Build history of the part. All positions in model axes, mm. Give positions to 0.01 mm unless a question says otherwise; leave off trailing zeros. Order: outer loops, then holes, each group sorted by start corner. A loop starts at its lowest first (then second) coordinate and runs counter-clockwise, first axis right, second up. Notation, with made-up numbers: (53, -13.5) - (58, -13.5) arc R12 cw to (58, 6.5) - close; hole circle Ø10 at (-29, 23.25). An arc over 180 degrees is marked (long way). Answer in a Markdown table with one row per item.
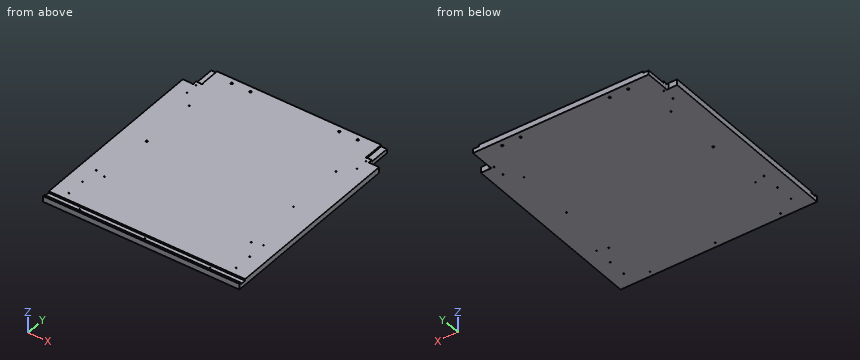
```python
from build123d import *

# Parameters (mm, degrees)
CABBACK_THICKNESS_DEPTH = 17.78
SKETCH4_R               = 3.175000003
SKETCH4_R_2             = 3.175000002
CUT_EXTRUDE1_DEPTH      = 17.78
SKETCH6_R               = 1.5875
SKETCH6_R_2             = 1.587500002
SKETCH6_R_3             = 2.777849083
CUT_EXTRUDE3_DEPTH      = 17.78
CABBACK_LEDGECUTS_W     = 17.78
CABBACK_LEDGECUTS_H     = 63.5
LEDGECUTS_DEPTH_DEPTH   = 5.08
SKETCH7_R               = 3.302
SKETCH7_R_2             = 3.302000002
CUT_EXTRUDE4_DEPTH      = 5.08
SKETCH9_R               = 3.175
CUT_EXTRUDE5_DEPTH      = 17.78


with BuildPart() as part:
    # CabBack_Outline → CabBack_Thickness (new body)
    with BuildSketch(Plane.XY):
        Polygon((10806.641666666, -6342.0625), (11409.891666666, -6342.0625), (11409.891666666, -5755.3225), (11378.141666665, -5755.3225), (11378.141666665, -5679.1225), (10838.391666667, -5679.1225), (10838.391666667, -5755.3225), (10806.641666666, -5755.3225), align=None)
    extrude(amount=-CABBACK_THICKNESS_DEPTH)

    # Sketch4 → Cut-Extrude1 (cut)
    with BuildSketch(Plane.XY):
        with Locations((11380.386730695, -5753.07743597)):
            Circle(SKETCH4_R)
        with Locations((10836.146602637, -5753.07743597)):
            Circle(SKETCH4_R_2)
    extrude(amount=-CUT_EXTRUDE1_DEPTH, mode=Mode.SUBTRACT)

    # Sketch6 → Cut-Extrude3 (cut)
    with BuildSketch(Plane.XY):
        with Locations((10851.409166666, -6294.4375)):
            Circle(SKETCH6_R)
        with Locations((10908.241666666, -6326.8225)):
            Circle(SKETCH6_R)
        with Locations((11108.266666666, -6326.8225)):
            Circle(SKETCH6_R)
        with Locations((11308.291666666, -6326.8225)):
            Circle(SKETCH6_R)
        with Locations((11365.124166666, -6294.4375)):
            Circle(SKETCH6_R)
        with Locations((11365.124166666, -6237.2875)):
            Circle(SKETCH6_R)
        with Locations((11333.691666666, -6188.3925)):
            Circle(SKETCH6_R)
        with Locations((11365.124166666, -6180.1375)):
            Circle(SKETCH6_R)
        with Locations((11333.691666666, -6010.5925)):
            Circle(SKETCH6_R)
        with Locations((11333.691666666, -5832.7925)):
            Circle(SKETCH6_R)
        with Locations((11369.251666663, -5793.344238991)):
            Circle(SKETCH6_R_2)
        with Locations((11369.251666663, -5755.236838581)):
            Circle(SKETCH6_R_2)
        with Locations((10847.281666666, -5755.236838581)):
            Circle(SKETCH6_R)
        with Locations((10847.281666666, -5793.344238991)):
            Circle(SKETCH6_R)
        with Locations((10882.841666666, -6010.5925)):
            Circle(SKETCH6_R_3)
        with Locations((10851.409166666, -6180.1375)):
            Circle(SKETCH6_R)
        with Locations((10882.841666666, -6188.3925)):
            Circle(SKETCH6_R)
        with Locations((10851.409166666, -6237.2875)):
            Circle(SKETCH6_R)
        with Locations((10882.841666666, -5832.7925)):
            Circle(SKETCH6_R)
    extrude(amount=-CUT_EXTRUDE3_DEPTH, mode=Mode.SUBTRACT)

    # CabBack_LedgeCuts → LedgeCuts_Depth (cut)
    with BuildSketch(Plane.XY):
        Polygon((11108.266666666, -6317.9325), (10806.641666666, -6317.9325), (10806.641666666, -6335.7125), (11409.891666666, -6335.7125), (11409.891666666, -6317.9325), align=None)
        with Locations((10847.281666667, -5710.8725)):
            Rectangle(CABBACK_LEDGECUTS_W, CABBACK_LEDGECUTS_H)
        with Locations((11369.251666665, -5710.8725)):
            Rectangle(CABBACK_LEDGECUTS_W, CABBACK_LEDGECUTS_H)
    extrude(amount=-LEDGECUTS_DEPTH_DEPTH, mode=Mode.SUBTRACT)

    # Sketch7 → Cut-Extrude4 (cut)
    with BuildSketch(Plane.XY):
        with Locations((10853.926602637, -5740.37743597)):
            Circle(SKETCH7_R)
        with Locations((11362.606730695, -5740.37743597)):
            Circle(SKETCH7_R_2)
    extrude(amount=-CUT_EXTRUDE4_DEPTH, mode=Mode.SUBTRACT)

    # Sketch9 → Cut-Extrude5 (cut)
    with BuildSketch(Plane.XY):
        with Locations((10914.541654066, -5697.2299822)):
            Circle(SKETCH9_R)
        with Locations((10971.741666666, -5697.2299822)):
            Circle(SKETCH9_R)
        with Locations((11244.741654066, -5697.2299822)):
            Circle(SKETCH9_R)
        with Locations((11301.941666666, -5697.2299822)):
            Circle(SKETCH9_R)
    extrude(amount=-CUT_EXTRUDE5_DEPTH, mode=Mode.SUBTRACT)


solid = part.part
```
1. Cut at A-A on y = -5729. Write the cut outline in (x, z), and give its area (3 significant figures).
Check result:
| item | result |
|---|---|
| outline | (10838.39, -17.78) - (11378.14, -17.78) - (11378.14, -5.08) - (11360.36, -5.08) - (11360.36, 0) - (10856.17, 0) - (10856.17, -5.08) - (10838.39, -5.08) - close |
| area | 9,420 mm² |
2. Probe line 1 (Y direction, x = 10992, z = -4.25); line 2 (X direction, y = -6295, z = -3.75); line 3 (Y direction, x = 11301.5, z = -3.5). List the from-to ranges inside material, lowest first.
Check result:
| item | result |
|---|---|
| line 1 | y = -6342.06 to -6335.71, -6317.93 to -5679.12 |
| line 2 | x = 10806.64 to 10849.92, 10852.89 to 11363.64, 11366.61 to 11409.89 |
| line 3 | y = -6342.06 to -6335.71, -6317.93 to -5700.37, -5694.09 to -5679.12 |
3. Drop flat-ended pins along their axis: P1, Ø1, axis at y = -5753, z = -8, coming from the -X side; P2, Ø4, axis at x = 11108.27, y = -6326.82, coming from the +Z side. Give the stop position or say it passes through.
Check result:
| item | result |
|---|---|
| P1 | stops at x = 10839.27 |
| P2 | stops at z = -5.08 |
